Geometry: final body of the model. Coordinates: model frame, mm. Face numbers are marked on the shaded views. A direction names the side the tool comes from. Give positions to 0.01 mm unless a question says otherwise; leave off trailing zeros. Write each loop counter-clockwise with the first axis right and the second up, starting at its lowest first coordinate (ties: lowest second). Pieces come first, ordered by that corner, then holes.
Q1. Reachability of the marked faces 1, 2 and 3 from +Z, -Z, +X, -X, +Y, -Y: full face, straight path, thin tool, end or side. Return the list, or none.
Q2. Cut plane D-D on z = 18. Count the separate pieces of the cut face and the enclosed holes in it, plus the area to 3 significant figures.
Q3. Pin query (flat end, axial travel): pin 1 (5.5 mm diameter, centred on x = 177.88, y = 43.66, fed in from -Z); pin 2 (4 mm diameter, centred on x = 27, y = -166.5, fed in from +Z); pin 3 (2 mm diameter, centred on y = -206.5, z = 22.5, fed in from -X). Return the tip coordinate at first contact, or that it passes through.
Q4. Cut plane C-C on y = 4. Return the cut outline in (x, z).
Q5. Cut plane B-B on x = 61. Return the cut outline in (y, z) (1 decimal).
Q6. Draft query along X for the marked faces 4, 5, 6 and 7. Return one class per face: pulls with the +X half, pulls with the -X half, needs draft (parallel to the pull), parting line crosses it, or undercut.
Q7. Line query: L1, parallel to X at y = -57.5, z = 46.5; L2, parallel to Y at x = 93, z = 36.5; L3, parallel to Y at x = 84, z = 24. Output: solid intervals per line, ascending.
Q8. Cut plane A-A on y = -143. Return the cut outline in (x, z) (1 decimal), plus the area to 3 significant figures.
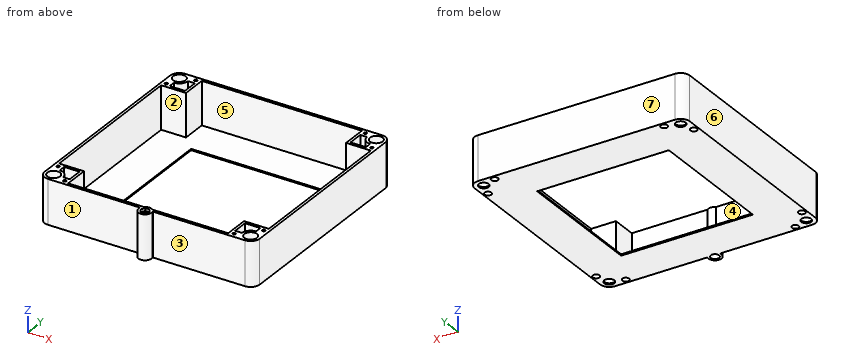
```python
from build123d import *

# Parameters (mm, degrees)
F0_R      = 1.7272
F0_R_2    = 5.9124977
F0_W      = 155.575
F0_H      = 155.575
F1_DEPTH  = 1.5875
F2_R      = 1.7272
F2_R_2    = 7.5
F3_DEPTH  = 50.8
F4_R      = 3.96875
F5_DEPTH  = 25.4
F6_R      = 10.6749977
F9_DEPTH  = 3.175
F7_R      = 4.9641200318
F10_DEPTH = 25.4


with BuildPart() as f1:
    # F0 (on Top) → F1 (new body)
    with BuildSketch(Plane.XY):
        with BuildLine():
            Line((204.7875, -204.7875), (204.7875, 49.2125))
            Line((204.7875, 49.2125), (-49.2125, 49.2125))
            Line((-49.2125, 49.2125), (-49.2125, -204.7875))
            Line((-49.2125, -204.7875), (70.0918461, -204.7875))
            Line((70.0918461, -204.7875), (75.9769233055, -204.7875))
            ThreePointArc((75.9769233055, -204.7875), (77.7875, -204.2206482), (79.5980766945, -204.7875))
            Line((79.5980766945, -204.7875), (85.4831539, -204.7875))
            Line((85.4831539, -204.7875), (204.7875, -204.7875))
        make_face()
        with Locations((-22.3062546, -199.23125)):
            Circle(F0_R, mode=Mode.SUBTRACT)
        with Locations((-38.5375023, -194.1125023)):
            Circle(F0_R_2, mode=Mode.SUBTRACT)
        with Locations((-43.65625, -177.8812546)):
            Circle(F0_R, mode=Mode.SUBTRACT)
        with Locations((177.8812546, -199.23125)):
            Circle(F0_R, mode=Mode.SUBTRACT)
        with Locations((194.1125023, -194.1125023)):
            Circle(F0_R_2, mode=Mode.SUBTRACT)
        with Locations((199.23125, -177.8812546)):
            Circle(F0_R, mode=Mode.SUBTRACT)
        with Locations((-43.65625, 22.3062546)):
            Circle(F0_R, mode=Mode.SUBTRACT)
        with Locations((-38.5375023, 38.5375023)):
            Circle(F0_R_2, mode=Mode.SUBTRACT)
        with Locations((-22.3062546, 43.65625)):
            Circle(F0_R, mode=Mode.SUBTRACT)
        with Locations((77.7875, -77.7875)):
            Rectangle(F0_W, F0_H, mode=Mode.SUBTRACT)
        with Locations((199.23125, 22.3062546)):
            Circle(F0_R, mode=Mode.SUBTRACT)
        with Locations((177.8812546, 43.65625)):
            Circle(F0_R, mode=Mode.SUBTRACT)
        with Locations((194.1125023, 38.5375023)):
            Circle(F0_R_2, mode=Mode.SUBTRACT)
        with BuildLine():
            Line((85.4831539, -207.3956482), (85.4831539, -204.7875))
            Line((85.4831539, -204.7875), (79.5980766945, -204.7875))
            ThreePointArc((79.5980766945, -204.7875), (80.6007904227, -205.9239070552), (80.9625, -207.3956482))
            ThreePointArc((80.9625, -207.3956482), (76.3157588552, -210.2089386227), (75.9769233055, -204.7875))
            Line((75.9769233055, -204.7875), (70.0918461, -204.7875))
            Line((70.0918461, -204.7875), (70.0918461, -207.3956482))
            ThreePointArc((70.0918461, -207.3956482), (77.7875, -215.0913021), (85.4831539, -207.3956482))
        make_face()
    extrude(amount=F1_DEPTH)

    # F2 (on face) → F3 (join)
    with BuildSketch(Plane.XY.offset(1.5875)):
        with BuildLine():
            Line((204.7875, -204.7875), (204.7875, 49.2125))
            Line((204.7875, 49.2125), (-49.2125, 49.2125))
            Line((-49.2125, 49.2125), (-49.2125, -204.7875))
            Line((-49.2125, -204.7875), (70.0918461, -204.7875))
            Line((70.0918461, -204.7875), (75.9769233055, -204.7875))
            ThreePointArc((75.9769233055, -204.7875), (77.7875, -204.2206482), (79.5980766945, -204.7875))
            Line((79.5980766945, -204.7875), (85.4831539, -204.7875))
            Line((85.4831539, -204.7875), (204.7875, -204.7875))
        make_face()
        with Locations((-22.3062546, -199.23125)):
            Circle(F2_R, mode=Mode.SUBTRACT)
        with Locations((-38.5375023, -194.1125023)):
            Circle(F2_R_2, mode=Mode.SUBTRACT)
        with BuildLine():
            Line((-38.1, -175.5000046), (-19.9250046, -175.5000046))
            Line((-19.9250046, -175.5000046), (-19.9250046, -193.675))
            Line((-19.9250046, -193.675), (-27.871473628, -193.675))
            ThreePointArc((-27.871473628, -193.675), (-30.9891390372, -186.5641390372), (-38.1, -183.446473628))
            Line((-38.1, -183.446473628), (-38.1, -175.5000046))
        make_face(mode=Mode.SUBTRACT)
        with Locations((-43.65625, -177.8812546)):
            Circle(F2_R, mode=Mode.SUBTRACT)
        with Locations((177.8812546, -199.23125)):
            Circle(F2_R, mode=Mode.SUBTRACT)
        with BuildLine():
            Line((175.5000046, -193.675), (175.5000046, -175.5000046))
            Line((175.5000046, -175.5000046), (193.675, -175.5000046))
            Line((193.675, -175.5000046), (193.675, -183.446473628))
            ThreePointArc((193.675, -183.446473628), (186.5641390372, -186.5641390372), (183.446473628, -193.675))
            Line((183.446473628, -193.675), (175.5000046, -193.675))
        make_face(mode=Mode.SUBTRACT)
        with Locations((194.1125023, -194.1125023)):
            Circle(F2_R_2, mode=Mode.SUBTRACT)
        with Locations((199.23125, -177.8812546)):
            Circle(F2_R, mode=Mode.SUBTRACT)
        with Locations((-43.65625, 22.3062546)):
            Circle(F2_R, mode=Mode.SUBTRACT)
        with BuildLine():
            Line((-19.9250046, 38.1), (-19.9250046, 19.9250046))
            Line((-19.9250046, 19.9250046), (-38.1, 19.9250046))
            Line((-38.1, 19.9250046), (-38.1, 27.871473628))
            ThreePointArc((-38.1, 27.871473628), (-30.9891390372, 30.9891390372), (-27.871473628, 38.1))
            Line((-27.871473628, 38.1), (-19.9250046, 38.1))
        make_face(mode=Mode.SUBTRACT)
        with Locations((-38.5375023, 38.5375023)):
            Circle(F2_R_2, mode=Mode.SUBTRACT)
        with Locations((-22.3062546, 43.65625)):
            Circle(F2_R, mode=Mode.SUBTRACT)
        Polygon((-16.7500046, 46.0375), (172.3250046, 46.0375), (172.3250046, 16.7500046), (201.6125, 16.7500046), (201.6125, -172.3250046), (172.3250046, -172.3250046), (172.3250046, -201.6125), (82.8647321047, -201.6125), (72.7102678953, -201.6125), (-16.7500046, -201.6125), (-16.7500046, -172.3250046), (-46.0375, -172.3250046), (-46.0375, 16.7500046), (-16.7500046, 16.7500046), align=None, mode=Mode.SUBTRACT)
        with BuildLine():
            Line((193.675, 19.9250046), (175.5000046, 19.9250046))
            Line((175.5000046, 19.9250046), (175.5000046, 38.1))
            Line((175.5000046, 38.1), (183.446473628, 38.1))
            ThreePointArc((183.446473628, 38.1), (186.5641390372, 30.9891390372), (193.675, 27.871473628))
            Line((193.675, 27.871473628), (193.675, 19.9250046))
        make_face(mode=Mode.SUBTRACT)
        with Locations((199.23125, 22.3062546)):
            Circle(F2_R, mode=Mode.SUBTRACT)
        with Locations((177.8812546, 43.65625)):
            Circle(F2_R, mode=Mode.SUBTRACT)
        with Locations((194.1125023, 38.5375023)):
            Circle(F2_R_2, mode=Mode.SUBTRACT)
        with BuildLine():
            Line((85.4831539, -207.3956482), (85.4831539, -204.7875))
            Line((85.4831539, -204.7875), (79.5980766945, -204.7875))
            ThreePointArc((79.5980766945, -204.7875), (80.6007904227, -205.9239070552), (80.9625, -207.3956482))
            ThreePointArc((80.9625, -207.3956482), (76.3157588552, -210.2089386227), (75.9769233055, -204.7875))
            Line((75.9769233055, -204.7875), (70.0918461, -204.7875))
            Line((70.0918461, -204.7875), (70.0918461, -207.3956482))
            ThreePointArc((70.0918461, -207.3956482), (77.7875, -215.0913021), (85.4831539, -207.3956482))
        make_face()
        with BuildLine():
            Line((72.7102678953, -201.6125), (82.8647321047, -201.6125))
            ThreePointArc((82.8647321047, -201.6125), (77.7875, -199.6999943), (72.7102678953, -201.6125))
        make_face()
    extrude(amount=F3_DEPTH)

    # F4 (on face) → F5 (cut)
    with BuildSketch(Plane(origin=(0, 0, 0), x_dir=(1, 0, 0), z_dir=(0, 0, -1))):
        with Locations((-43.65625, -22.3062546)):
            Circle(F4_R)
        with Locations((-22.3062546, -43.65625)):
            Circle(F4_R)
        with Locations((-43.65625, 177.8812546)):
            Circle(F4_R)
        with Locations((-22.3062546, 199.23125)):
            Circle(F4_R)
        with Locations((199.23125, 177.8812546)):
            Circle(F4_R)
        with Locations((177.8812546, 199.23125)):
            Circle(F4_R)
        with Locations((177.8812546, -43.65625)):
            Circle(F4_R)
        with Locations((199.23125, -22.3062546)):
            Circle(F4_R)
    extrude(amount=-F5_DEPTH, mode=Mode.SUBTRACT)

    # F6
    f6_edges = [f1.edges().sort_by_distance(p)[0] for p in [
        (204.7875, 49.2125, 26.19375),
        (204.7875, -204.7875, 26.19375),
        (-49.2125, -204.7875, 26.19375),
        (-49.2125, 49.2125, 26.19375),
    ]]
    fillet(f6_edges, radius=F6_R)

    # F8 (on face) → F9 (cut)
    with BuildSketch(Plane.XY.offset(52.3875)):
        Polygon((75.1774992539, -211.9163021), (80.3975007461, -211.9163021), (83.0075014922, -207.3956482), (80.3975007461, -202.8749943), (75.1774992539, -202.8749943), (72.5674985078, -207.3956482), align=None)
    extrude(amount=-F9_DEPTH, mode=Mode.SUBTRACT)

    # F7 (on face) → F10 (cut)
    with BuildSketch(Plane(origin=(0, 0, 0), x_dir=(1, 0, 0), z_dir=(0, 0, -1))):
        with Locations((77.7875, 207.3956482)):
            Circle(F7_R)
    extrude(amount=-F10_DEPTH, mode=Mode.SUBTRACT)


solid = f1.part
```
Data:
1. face 1: +Z, -Z, -X, -Y
1. face 2: +Z
1. face 3: +Z, -Z, +X, -Y
2. separate pieces: 1
2. enclosed holes: 18
2. area: 4,490 mm2
3. pin 1: stops at z = 25.4
3. pin 2: stops at z = 1.59
3. pin 3: stops at x = 70.09
4. outline: (-49.21, 0) - (204.79, 0) - (204.79, 52.39) - (201.61, 52.39) - (201.61, 1.59) - (-46.04, 1.59) - (-46.04, 52.39) - (-49.21, 52.39) - close
5. outline: (-204.8, 0) - (-155.6, 0) - (-155.6, 1.6) - (-201.6, 1.6) - (-201.6, 52.4) - (-204.8, 52.4) - close; (0, 0) - (49.2, 0) - (49.2, 52.4) - (46, 52.4) - (46, 1.6) - (0, 1.6) - close
6. face 4: undercut
6. face 5: undercut
6. face 6: pulls with the -X half
6. face 7: needs draft
7. L1: x = -49.21 to -46.04, 201.61 to 204.79
7. L2: y = -204.79 to -201.61, 46.04 to 49.21
7. L3: y = -211.94 to -201.61, 46.04 to 49.21
8. outline: (-49.2, 0) - (0, 0) - (0, 1.6) - (-46, 1.6) - (-46, 52.4) - (-49.2, 52.4) - close; (155.6, 0) - (204.8, 0) - (204.8, 52.4) - (201.6, 52.4) - (201.6, 1.6) - (155.6, 1.6) - close
8. area: 479 mm2
